Job drawing, mm, ordinate dimensions from the low corner. One solid piece. Coordinates: 2 decimals unless noted, no trailing zeros. Order: outer loops, then holes, each group sorted by start corner. A loop starts at its lowest first (then second) coordinate and runs counter-clockwise, first axis right, second up. Notation, with made-up numbers: (-25, 54.25) - (-12, 54.25) arc R37 cw to (-12, 92.25) - close; hole circle Ø5 at (70, 55.5). An arc over 180 degrees is marked (long way). Use a Markdown table: item, result. Add a question column.
1) Drop flat-ended pins along their axis: P1, Ø1, axis at y = 0.5, z = 14, coming from the +X side; P2, Ø1, axis at x = 5, y = 1, coming from the -Z side (1 decimal). Give the stop position or say it passes through.
2) Saw through at B-B on z = 20. List the corners of the cut face in (x, y) (1 decimal).
3) Wall check: L1, parallel to X at y = 2.3, z = 15 (1 decimal); L2, parallel to Z at x = 21.5, y = 2.15 (1 decimal); L3, parallel to Z at x = 21, y = 1.9. Give the ranges that are in metal, low to high. Write a range as [from, to].
4) Saw through at A-A on y = 1.5. Count the separate pieces of the cut face and the enclosed holes in it, then the cut area to 3 significant figures.
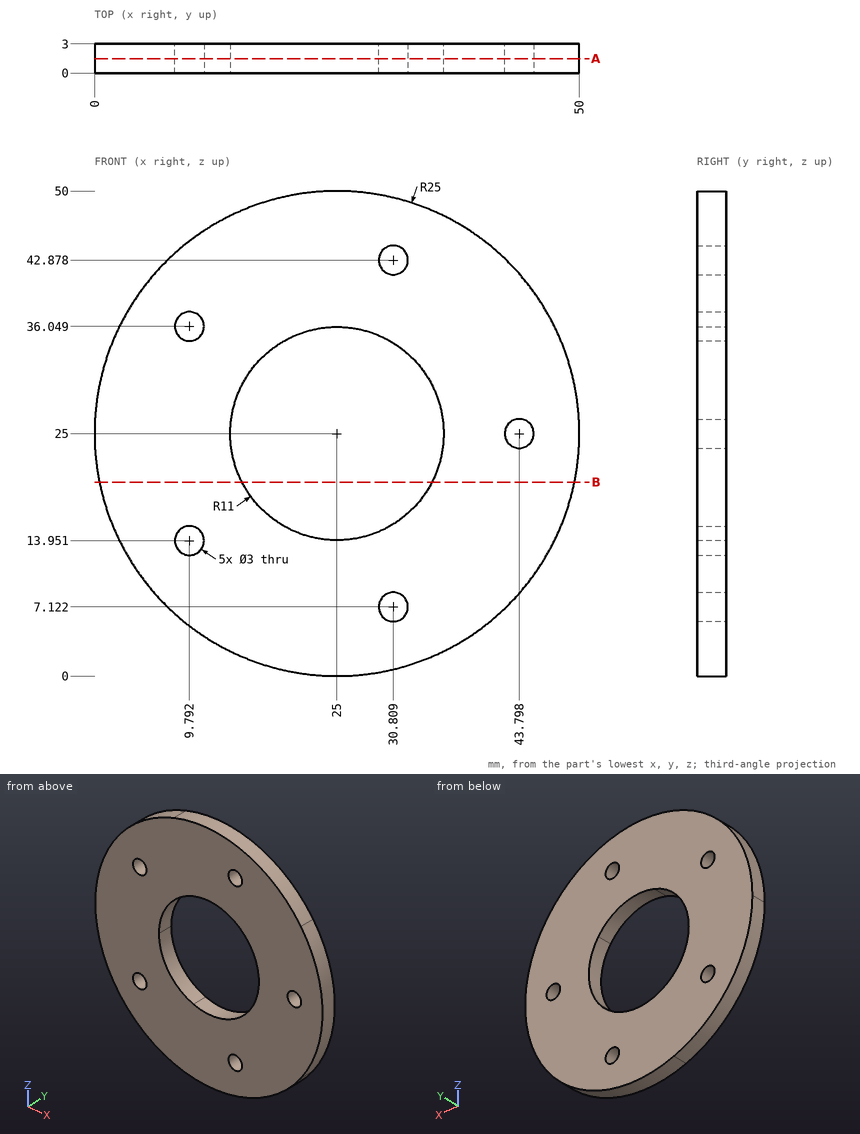
Results are:
| question | item | result |
|---|---|---|
| 1 | P1 | x = 47.69 |
| 1 | P2 | z = 9.4 |
| 2 | outline | (0.5, 0) - (15.2, 0) - (15.2, 3) - (0.5, 3) - close; (34.8, 0) - (49.5, 0) - (49.5, 3) - (34.8, 3) - close |
| 3 | L1 | [2.1, 8.7], [10.9, 20.4], [29.6, 47.9] |
| 3 | L2 | [0.2, 14.6], [35.4, 49.8] |
| 3 | L3 | [0.32, 14.75], [35.25, 49.68] |
| 4 | separate pieces | 1 |
| 4 | enclosed holes | 6 |
| 4 | area | 1,550 mm2 |
